Verification items for the finished model (mm, model axes). Round coordinates to 2 decimals unless told otherwise and drop trailing zeros. Write each loop counter-clockwise with the first axis right and the second up, starting at its lowest first coordinate (ties: lowest second). Pieces come first, ordered by that corner, then holes. Notation, with made-up numbers: (24.5, 74.25) - (33.5, 74.25) arc R11 ccw to (33.5, 95.25) - close; hole circle Ø5 at (-15.5, 57.5). An arc over 180 degrees is marked (long way). Answer as a JSON object with one key per item and string values. Group by question number.
1) Go/stop test with flat-tipped pins: pin 1 Ø3 at (x, z) = (-13.11, 6.18) entering from +Y; pin 2 Ø12 at (x, z) = (0, -10.5) entering from -Y. Record where each tip stops, or that it passes through.
2) Thickness scan on line 1 (X direction, y = 1.15, z = -12.75); line 2 (Z direction, x = 4, y = 1.45); line 3 (X direction, y = 0.8, z = 13.5). Record the ranges inside material, lowest first.
3) Section check C-C (x = -5). Enter the section's corners in (y, z).
4) Section check D-D (y = 0.4). State how many separate pieces and enclosed holes the cut face has, then the cut area to 3 significant figures.
5) Section check B-B (x = -18). Enter the section's corners in (y, z), then the cut area to 3 significant figures.
6) Section check A-A (z = 3). Enter the section's corners in (x, y), then the cut area to 3 significant figures.
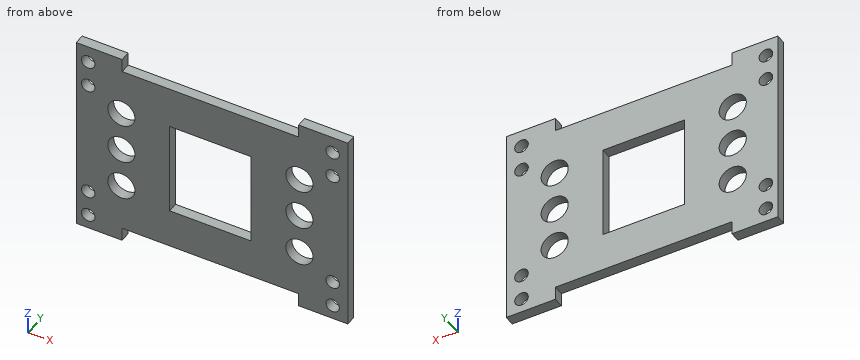
```python
from build123d import *

# Parameters (mm, degrees)
TOP_PLATE_2_SKETCH_R   = 1
TOP_PLATE_2_SKETCH_R_2 = 2
TOP_PLATE_2_SKETCH_W   = 12
TOP_PLATE_2_SKETCH_H   = 14
TOP_PLATE_2_DEPTH      = 1.5


with BuildPart() as part:
    # Top Plate 2 Sketch → Top Plate 2 (new body)
    with BuildSketch(Plane(origin=(0, 0, 0), x_dir=(1, 0, 0), z_dir=(0, 1, 0))):
        Polygon((-13, 14.817316164), (-19.756421551, 14.817316164), (-19.756421551, -15.182683836), (-13, -15.182683836), (-13, -13.182683836), (13, -13.182683836), (13, -15.182683836), (20.243578449, -15.182683836), (20.243578449, 14.817316164), (13, 14.817316164), (13, 12.817316164), (-13, 12.817316164), align=None)
        with Locations(Location((-18, -12.682683836, 0), (0, 0, 270))):
            Circle(TOP_PLATE_2_SKETCH_R, mode=Mode.SUBTRACT)
        with Locations(Location((-18, -8.782683836, 0), (0, 0, 270))):
            Circle(TOP_PLATE_2_SKETCH_R, mode=Mode.SUBTRACT)
        with Locations(Location((-13.113273082, -6.182683836, 0), (0, 0, 270))):
            Circle(TOP_PLATE_2_SKETCH_R_2, mode=Mode.SUBTRACT)
        with Locations(Location((18, -12.682683836, 0), (0, 0, 270))):
            Circle(TOP_PLATE_2_SKETCH_R, mode=Mode.SUBTRACT)
        with Locations(Location((18, -8.782683836, 0), (0, 0, 270))):
            Circle(TOP_PLATE_2_SKETCH_R, mode=Mode.SUBTRACT)
        with Locations(Location((13.113273082, -6.182683836, 0), (0, 0, 270))):
            Circle(TOP_PLATE_2_SKETCH_R_2, mode=Mode.SUBTRACT)
        with Locations(Location((-13.113273082, -0.182683836, 0), (0, 0, 270))):
            Circle(TOP_PLATE_2_SKETCH_R_2, mode=Mode.SUBTRACT)
        with Locations(Location((-13.113273082, 5.817316164, 0), (0, 0, 270))):
            Circle(TOP_PLATE_2_SKETCH_R_2, mode=Mode.SUBTRACT)
        Rectangle(TOP_PLATE_2_SKETCH_W, TOP_PLATE_2_SKETCH_H, mode=Mode.SUBTRACT)
        with Locations(Location((-18, 8.782683836, 0), (0, 0, 270))):
            Circle(TOP_PLATE_2_SKETCH_R, mode=Mode.SUBTRACT)
        with Locations(Location((-18, 12.682683836, 0), (0, 0, 270))):
            Circle(TOP_PLATE_2_SKETCH_R, mode=Mode.SUBTRACT)
        with Locations(Location((13.113273082, -0.182683836, 0), (0, 0, 270))):
            Circle(TOP_PLATE_2_SKETCH_R_2, mode=Mode.SUBTRACT)
        with Locations(Location((13.113273082, 5.817316164, 0), (0, 0, 270))):
            Circle(TOP_PLATE_2_SKETCH_R_2, mode=Mode.SUBTRACT)
        with Locations(Location((18, 8.782683836, 0), (0, 0, 270))):
            Circle(TOP_PLATE_2_SKETCH_R, mode=Mode.SUBTRACT)
        with Locations(Location((18, 12.682683836, 0), (0, 0, 270))):
            Circle(TOP_PLATE_2_SKETCH_R, mode=Mode.SUBTRACT)
    extrude(amount=TOP_PLATE_2_DEPTH)


solid = part.part
```
Returned:
{
 "1": {"pin 1": "through", "pin 2": "y = 0"},
 "2": {"line 1": "-19.76 to -19, -17 to 17, 19 to 20.24", "line 2": "-12.82 to -7, 7 to 13.18", "line 3": "-19.76 to -18.58, -17.42 to -13, 13 to 17.42, 18.58 to 20.24"},
 "3": {"outline": "(0, -12.82) - (1.5, -12.82) - (1.5, -7) - (0, -7) - close; (0, 7) - (1.5, 7) - (1.5, 13.18) - (0, 13.18) - close"},
 "4": {"separate pieces": "1", "enclosed holes": "15", "area": "827 mm2"},
 "5": {"outline": "(0, -14.82) - (1.5, -14.82) - (1.5, -13.68) - (0, -13.68) - close; (0, -11.68) - (1.5, -11.68) - (1.5, -9.78) - (0, -9.78) - close; (0, -7.78) - (1.5, -7.78) - (1.5, 7.78) - (0, 7.78) - close; (0, 9.78) - (1.5, 9.78) - (1.5, 11.68) - (0, 11.68) - close; (0, 13.68) - (1.5, 13.68) - (1.5, 15.18) - (0, 15.18) - close", "area": "33.0 mm2"},
 "6": {"outline": "(-19.76, 0) - (-6, 0) - (-6, 1.5) - (-19.76, 1.5) - close; (6, 0) - (20.24, 0) - (20.24, 1.5) - (6, 1.5) - close", "area": "42.0 mm2"}
}
